from build123d import *

# Parameters (mm, degrees)
SKETCH_1_W          = 106
SKETCH_1_H          = 40
EXTRUDE_1_DEPTH     = 1.5
SKETCH_5_W          = 106
SKETCH_5_H          = 36.5
EXTRUDE_4_DEPTH     = 1.5
SKETCH_6_W          = 106
SKETCH_6_H          = 66
EXTRUDE_5_DEPTH     = 1.5
EXTRUDE_6_DEPTH     = 10
EXTRUDE_7_DEPTH     = 46.5
SKETCH_11_W         = 8.1
SKETCH_11_H         = 11.2
CUT_EXTRUDE_1_DEPTH = 1.5
SKETCH_12_W         = 11.1
SKETCH_12_H         = 14.2
SKETCH_12_W_2       = 8.1
SKETCH_12_H_2       = 11.2
EXTRUDE_8_DEPTH     = 10
SKETCH_13_W         = 78
SKETCH_13_H         = 26
CUT_EXTRUDE_2_DEPTH = 1.5


with BuildPart() as part:
    # 草图1 → 凸台-拉伸1 (new body)
    with BuildSketch(Plane.XY):
        with Locations((53, -20)):
            Rectangle(SKETCH_1_W, SKETCH_1_H)
    extrude(amount=EXTRUDE_1_DEPTH)

    # 草图5 → 凸台-拉伸4 (add)
    with BuildSketch(Plane.XZ.offset(40)):
        with Locations((53, 18.25)):
            Rectangle(SKETCH_5_W, SKETCH_5_H)
    extrude(amount=EXTRUDE_4_DEPTH)

    # 草图6 → 凸台-拉伸5 (add)
    with BuildSketch(Plane.XY.offset(36.5)):
        with Locations((53, -73)):
            Rectangle(SKETCH_6_W, SKETCH_6_H)
    extrude(amount=EXTRUDE_5_DEPTH)

    # 草图7 → 凸台-拉伸6 (add)
    with BuildSketch(Plane(origin=(0, 0, 0), x_dir=(-1, 0, 0), z_dir=(0, 0, -1))):
        Polygon((-106, -41.5), (-106, 0), (0, 0), (0, -41.5), (-1.5, -41.5), (-1.5, -1.5), (-104.5, -1.5), (-104.5, -41.5), align=None)
    extrude(amount=EXTRUDE_6_DEPTH)

    # 草图8 → 凸台-拉伸7 (add)
    with BuildSketch(Plane(origin=(0, 0, 36.5), x_dir=(-1, 0, 0), z_dir=(0, 0, -1))):
        Polygon((-106, -41.5), (-106, -106), (0, -106), (0, -41.5), (-1.5, -41.5), (-1.5, -104.5), (-104.5, -104.5), (-104.5, -41.5), align=None)
    extrude(amount=EXTRUDE_7_DEPTH)

    # 草图11 → 切除-拉伸1 (cut)
    with BuildSketch(Plane.XY.offset(38)):
        Polygon((63.911237552, -74.99759487), (63.911237552, -75.99809487), (63.110437552, -75.99809487), (63.110437552, -79.09729487), (63.911237552, -79.09729487), (63.911237552, -84.89729487), (63.110437552, -84.89729487), (63.110437552, -87.99789487), (63.911237552, -87.99789487), (63.911237552, -88.99829487), (77.910537552, -88.99829487), (77.910537552, -87.99789487), (78.711337552, -87.99789487), (78.711337552, -84.89729487), (77.910537552, -84.89729487), (77.910537552, -79.09729487), (78.711337552, -79.09729487), (78.711337552, -75.99809487), (77.910537552, -75.99809487), (77.910537552, -74.99759487), align=None)
        Polygon((44.861237552, -74.99759487), (44.861237552, -75.99809487), (44.060437552, -75.99809487), (44.060437552, -79.09729487), (44.861237552, -79.09729487), (44.861237552, -84.89729487), (44.060437552, -84.89729487), (44.060437552, -87.99789487), (44.861237552, -87.99789487), (44.861237552, -88.99829487), (58.860537552, -88.99829487), (58.860537552, -87.99789487), (59.661337552, -87.99789487), (59.661337552, -84.89729487), (58.860537552, -84.89729487), (58.860537552, -79.09729487), (59.661337552, -79.09729487), (59.661337552, -75.99809487), (58.860537552, -75.99809487), (58.860537552, -74.99759487), align=None)
        Polygon((25.811237552, -74.99759487), (25.811237552, -75.99809487), (25.010537552, -75.99809487), (25.010537552, -79.09729487), (25.811237552, -79.09729487), (25.811237552, -84.89729487), (25.010537552, -84.89729487), (25.010537552, -87.99789487), (25.811237552, -87.99789487), (25.811237552, -88.99829487), (39.810537552, -88.99829487), (39.810537552, -87.99789487), (40.611337552, -87.99789487), (40.611337552, -84.89729487), (39.810537552, -84.89729487), (39.810537552, -79.09729487), (40.611337552, -79.09729487), (40.611337552, -75.99809487), (39.810537552, -75.99809487), (39.810537552, -74.99759487), align=None)
        Polygon((6.761187552, -74.99759487), (6.761187552, -75.99809487), (5.960547552, -75.99809487), (5.960547552, -79.09729487), (6.761187552, -79.09729487), (6.761187552, -84.89729487), (5.960547552, -84.89729487), (5.960547552, -87.99789487), (6.761187552, -87.99789487), (6.761187552, -88.99829487), (20.760737552, -88.99829487), (20.760737552, -87.99789487), (21.561337552, -87.99789487), (21.561337552, -84.89729487), (20.760737552, -84.89729487), (20.760737552, -79.09729487), (21.561337552, -79.09729487), (21.561337552, -75.99809487), (20.760737552, -75.99809487), (20.760737552, -74.99759487), align=None)
        Polygon((63.911237552, -55.94899487), (63.911237552, -56.94949487), (63.110437552, -56.94949487), (63.110437552, -60.04869487), (63.911237552, -60.04869487), (63.911237552, -65.84869487), (63.110437552, -65.84869487), (63.110437552, -68.94929487), (63.911237552, -68.94929487), (63.911237552, -69.94829487), (77.910537552, -69.94829487), (77.910537552, -68.94929487), (78.711337552, -68.94929487), (78.711337552, -65.84869487), (77.910537552, -65.84869487), (77.910537552, -60.04869487), (78.711337552, -60.04869487), (78.711337552, -56.94949487), (77.910537552, -56.94949487), (77.910537552, -55.94899487), align=None)
        Polygon((44.861237552, -55.94899487), (44.861237552, -56.94949487), (44.060437552, -56.94949487), (44.060437552, -60.04869487), (44.861237552, -60.04869487), (44.861237552, -65.84869487), (44.060437552, -65.84869487), (44.060437552, -68.94929487), (44.861237552, -68.94929487), (44.861237552, -69.94829487), (58.860537552, -69.94829487), (58.860537552, -68.94929487), (59.661337552, -68.94929487), (59.661337552, -65.84869487), (58.860537552, -65.84869487), (58.860537552, -60.04869487), (59.661337552, -60.04869487), (59.661337552, -56.94949487), (58.860537552, -56.94949487), (58.860537552, -55.94899487), align=None)
        Polygon((25.811237552, -55.94899487), (25.811237552, -56.94949487), (25.010537552, -56.94949487), (25.010537552, -60.04869487), (25.811237552, -60.04869487), (25.811237552, -65.84869487), (25.010537552, -65.84869487), (25.010537552, -68.94929487), (25.811237552, -68.94929487), (25.811237552, -69.94829487), (39.810537552, -69.94829487), (39.810537552, -68.94929487), (40.611337552, -68.94929487), (40.611337552, -65.84869487), (39.810537552, -65.84869487), (39.810537552, -60.04869487), (40.611337552, -60.04869487), (40.611337552, -56.94949487), (39.810537552, -56.94949487), (39.810537552, -55.94899487), align=None)
        Polygon((6.761187552, -55.94899487), (6.761187552, -56.94949487), (5.960547552, -56.94949487), (5.960547552, -60.04869487), (6.761187552, -60.04869487), (6.761187552, -65.84869487), (5.960547552, -65.84869487), (5.960547552, -68.94929487), (6.761187552, -68.94929487), (6.761187552, -69.94829487), (20.760737552, -69.94829487), (20.760737552, -68.94929487), (21.561337552, -68.94929487), (21.561337552, -65.84869487), (20.760737552, -65.84869487), (20.760737552, -60.04869487), (21.561337552, -60.04869487), (21.561337552, -56.94949487), (20.760737552, -56.94949487), (20.760737552, -55.94899487), align=None)
        with Locations((93.785079963, -74.54929487)):
            Rectangle(SKETCH_11_W, SKETCH_11_H)
    extrude(amount=-CUT_EXTRUDE_1_DEPTH, mode=Mode.SUBTRACT)

    # 草图12 → 凸台-拉伸8 (add)
    with BuildSketch(Plane(origin=(0, 0, 36.5), x_dir=(-1, 0, 0), z_dir=(0, 0, -1))):
        with Locations((-93.785079963, -74.54929487)):
            Rectangle(SKETCH_12_W, SKETCH_12_H)
        with Locations((-93.785079963, -74.54929487)):
            Rectangle(SKETCH_12_W_2, SKETCH_12_H_2, mode=Mode.SUBTRACT)
    extrude(amount=EXTRUDE_8_DEPTH)

    # 草图13 → 切除-拉伸2 (cut)
    with BuildSketch(Plane.XY.offset(1.5)):
        with Locations((52, -27)):
            Rectangle(SKETCH_13_W, SKETCH_13_H)
    extrude(amount=-CUT_EXTRUDE_2_DEPTH, mode=Mode.SUBTRACT)


solid = part.part
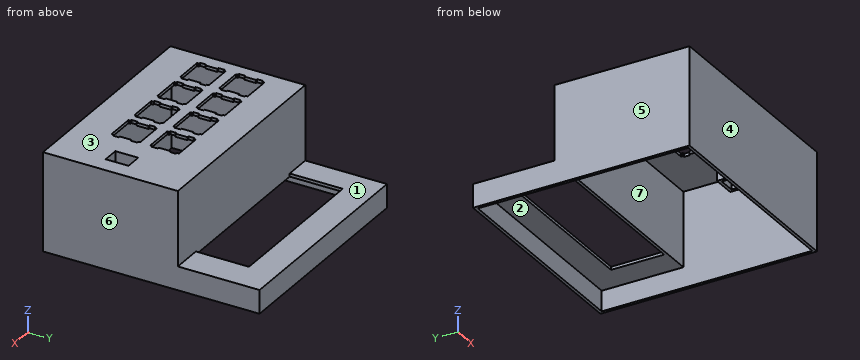
Geometry: final body of the model. Coordinates: model frame, mm. Face numbers are marked on the shaded views. A direction names the side the tool comes from. Give positions to 0.01 mm unless a question says otherwise; leave off trailing zeros. Write each loop counter-clockwise with the first axis right and the second up, starting at its lowest first coordinate (ties: lowest second). Pieces come first, ordered by that corner, then holes.
(1) Mould query, pull axis X, two halves, no side actions, for the marked faces 4, 5, 6 and 7. Classes: released by +X, released by -X, zero draft, split by the parting line, or undercut.
(2) Ray query, line 1 (Y direction, x = 93, z = 34.5); line 2 (X direction, y = -68.5, z = 30); line 3 (X direction, y = -74, z = -1). Return the intervals inside material, ascending.
(3) Cut plane D-D, the plane z = -1.5. Return loops of the section in (x, y), then the cut area to 3 significant figures.
(4) Cut plane B-B, the plane y = -83. Return loops of the section in (x, z), then the cut area to 3 significant figures.
(5) First-contact query: P1, Ø11, axis at x = 95, z = 29.5, coming from the +Y side; P2, Ø8, axis at y = -68, z = 10, coming from the -X side. Flat tips, straight axial feed; report the tip coordinate or a pass-through.
(6) Access query for the marked faces 1, 2 and 3. Directions: +Z, -Z, +X, -X, +Y, -Y. A direction counts if a zero-diameter tool reaches every point of the face in a straight line with its end or side. Return the directions, or none.
(7) Cut plane C-C, the plane x = 9. Return loops of the section in (y, z).
(8) Cut plane A-A, the plane z = 31.5. Return loops of the section in (x, y), then the cut area to 3 significant figures.
Values follow:
1. face 4: zero draft
1. face 5: released by -X
1. face 6: released by +X
1. face 7: undercut
2. line 1: y = -106 to -104.5, -81.65 to -80.15, -68.95 to -67.45, -41.5 to -40
2. line 2: x = 0 to 1.5, 88.24 to 99.34, 104.5 to 106
2. line 3: x = 0 to 1.5, 104.5 to 106
3. outline: (0, -106) - (106, -106) - (106, 0) - (0, 0) - close; hole (1.5, -104.5) - (104.5, -104.5) - (104.5, -1.5) - (1.5, -1.5) - close
3. area: 627 mm2
4. outline: (0, -10) - (1.5, -10) - (1.5, 36.5) - (6.76, 36.5) - (6.76, 38) - (0, 38) - close; (20.76, 36.5) - (25.81, 36.5) - (25.81, 38) - (20.76, 38) - close; (39.81, 36.5) - (44.86, 36.5) - (44.86, 38) - (39.81, 38) - close; (58.86, 36.5) - (63.91, 36.5) - (63.91, 38) - (58.86, 38) - close; (77.91, 36.5) - (104.5, 36.5) - (104.5, -10) - (106, -10) - (106, 38) - (77.91, 38) - close
4. area: 215 mm2
5. P1: stops at y = -40
5. P2: stops at x = 0
6. face 1: +Z, +X, -X, +Y
6. face 2: -Z
6. face 3: +Z, +X, -X, +Y, -Y
7. outline: (-106, -10) - (-104.5, -10) - (-104.5, 36.5) - (-89, 36.5) - (-89, 38) - (-106, 38) - close; (-75, 36.5) - (-69.95, 36.5) - (-69.95, 38) - (-75, 38) - close; (-55.95, 36.5) - (-41.5, 36.5) - (-41.5, 0) - (-1.5, 0) - (-1.5, -10) - (0, -10) - (0, 1.5) - (-40, 1.5) - (-40, 38) - (-55.95, 38) - close
8. outline: (0, -106) - (106, -106) - (106, -40) - (0, -40) - close; (88.24, -81.65) - (99.34, -81.65) - (99.34, -67.45) - (88.24, -67.45) - close; hole (1.5, -104.5) - (104.5, -104.5) - (104.5, -41.5) - (1.5, -41.5) - close; hole (89.74, -80.15) - (97.84, -80.15) - (97.84, -68.95) - (89.74, -68.95) - close
8. area: 574 mm2
